Input: part model. Units: mm. Frame: model coordinates. A direction names the side the tool comes from. Give positions to 0.01 mm unless a question says otherwise; leave off trailing zeros. Order: outer loops, then holes, each group sorted by start corner. A loop starts at its lowest first (then second) coordinate and runs counter-clockwise, first axis right, second up. Notation, with made-up numbers: M -10.75,82 L -0.75,82 A24 cw -0.75,105 Z; hole C 60.25,-22.5 d9. An arc over 180 degrees is marked long. Use a Markdown table: item, result.
from build123d import *

# Parameters (mm, degrees)
SKETCH1_W           = 66.294
SKETCH1_H           = 30.48
BOSS_EXTRUDE1_DEPTH = 3.175
SKETCH2_W           = 22.098
SKETCH2_H           = 6.35
BOSS_EXTRUDE2_DEPTH = 6.35
CAVITY1_START       = -5.08
CAVITY1_OUTLINE_W   = 5.207
CAVITY1_OUTLINE_H   = 6.35
CAVITY1_DEPTH       = 10.16


# Read off the part's stored shape, not the designer's step: Cavity1
with BuildPart() as part:
    # Sketch1 → Boss-Extrude1 (new, symmetric)
    with BuildSketch(Plane(origin=(0, 0, 0), x_dir=(1, 0, 0), z_dir=(0, 1, 0))):
        Rectangle(SKETCH1_W, SKETCH1_H)
    extrude(amount=BOSS_EXTRUDE1_DEPTH, both=True)

    # Sketch2 → Boss-Extrude2 (add)
    with BuildSketch(Plane(origin=(0, 3.175, 0), x_dir=(1, 0, 0), z_dir=(0, 1, 0))):
        with Locations((0, -18.415)):
            Rectangle(SKETCH2_W, SKETCH2_H)
    extrude(amount=-BOSS_EXTRUDE2_DEPTH)

    # Cavity1 outline → Cavity1 (cut)
    with BuildSketch(Plane.XY.offset(CAVITY1_START)):
        with Locations((30.5435, 0)):
            Rectangle(CAVITY1_OUTLINE_W, CAVITY1_OUTLINE_H)
        with Locations((-30.5435, 0)):
            Rectangle(CAVITY1_OUTLINE_W, CAVITY1_OUTLINE_H)
    extrude(amount=CAVITY1_DEPTH, mode=Mode.SUBTRACT)


solid = part.part
1) Material intervals for line 1 (X direction, y = 1, z = -0.5); line 2 (Z direction, x = 26.5, y = -0.5); line 3 (X direction, y = 2.25, z = 17), sorted ascending. Write a range as from..to.
Response values:
| item | result |
|---|---|
| line 1 | x = -27.94..27.94 |
| line 2 | z = -15.24..15.24 |
| line 3 | x = -11.05..11.05 |
2) Reachability of faces 5 (the face through (-11.049, 0, 18)), 6 (the face through (-31, 0, 5.08)), 7 (the face through (11.049, 0, 18)) from +Z, -Z, +X, -X, +Y, -Y: full face, straight path, thin tool, end or side. Return the list, or none.
Response values:
| item | result |
|---|---|
| face 5 | +Z, -X, +Y, -Y |
| face 6 | -X, +Y, -Y |
| face 7 | +Z, +X, +Y, -Y |
3) Mould query, pull axis Z, two halves, no side actions, for faces 1 (the face through (33.147, 0, 10)), 2 (the face through (0, 0, -15.24)), 3 (the face through (31, 0, -5.08)), 4 (the face through (27.94, 0, 0)). Classes: released by +Z, released by -Z, zero draft, split by the parting line, or undercut.
Response values:
| item | result |
|---|---|
| face 1 | zero draft |
| face 2 | released by -Z |
| face 3 | undercut |
| face 4 | undercut |
4) Cut plane C-C on z = 3. Return loops of the section in (x, y) (3 decimals).
Response values:
| item | result |
|---|---|
| outline | M -27.94,-3.175 L 27.94,-3.175 L 27.94,3.175 L -27.94,3.175 Z |
5) Cut plane A-A on y = -0.75. Return loops of the section in (x, z), and give its area (3 significant figures).
Response values:
| item | result |
|---|---|
| outline | M -33.15,-15.24 L 33.15,-15.24 L 33.15,-5.08 L 27.94,-5.08 L 27.94,5.08 L 33.15,5.08 L 33.15,15.24 L 11.05,15.24 L 11.05,21.59 L -11.05,21.59 L -11.05,15.24 L -33.15,15.24 L -33.15,5.08 L -27.94,5.08 L -27.94,-5.08 L -33.15,-5.08 Z |
| area | 2,060 mm² |
6) First-contact query: pin 1 Ø3 at (x, y) = (17.5, -0.5) entering from +Z. Flat tip, straight axial feed; report the tip coordinate or a pass-through.
Response values:
| item | result |
|---|---|
| pin 1 | stops at z = 15.24 |
7) Cut plane B-B on x = -12. Return loops of the section in (y, z) (3 decimals), and give its area (3 significant figures).
Response values:
| item | result |
|---|---|
| outline | M -3.175,-15.24 L 3.175,-15.24 L 3.175,15.24 L -3.175,15.24 Z |
| area | 194 mm² |
